Could you check a few things on this drawing? It's one solid part, dimensions in mm from its lowest x, y, z. A direction names the side the tool comes from. Give positions to 0.01 mm unless a question says otherwise; leave off trailing zeros. Loops run counter-clockwise (first coordinate to the right, second up) from the corner with the lowest first, then second, coordinate; pieces in that order, holes last. Notation, with made-up numbers: (-5.5, -7.5) - (45.5, -7.5) arc R23 cw to (45.5, 9.5) - close; hole circle Ø6 at (77, 37.25). An arc over 180 degrees is marked (long way). Return JSON: item names as keys, results as strings. Group by question number.
(1) If we section it at C-C (x = 27.1): Please give me the cut outline in (y, z), then the cut area to 3 significant figures.
(2) For P1, Ø1.5, axis at y = 12, z = 13, coming from the +X side; P2, Ø2.5, axis at y = 10.5, z = 11.5, coming from the +X side; P3, Ø18, axis at x = 63.5, y = 8.5, coming from the +Z side, each with a flat end and sliding along its axis, tell me the tip position at first contact or that it passes through.
(3) If we section it at D-D (z = 6): Please give me the cut outline in (x, y), then the cut area to 3 significant figures.
(4) If we mould it in two halves opening along X, with no side actions, what happens to the marked faces 1, 2 and 3? For each: released by +X, released by -X, zero draft, split by the parting line, or undercut.
(5) If we section it at B-B (z = 13): Please give me the cut outline in (x, y).
(6) On a 3-axis mill with a long thin cutter (end or side, diameter ignored), from which of +Z, -Z, +X, -X, +Y, -Y can I reach the whole of each face in a straight line? I mean the marked faces 4, 5 and 6. Say none if no direction works.
(7) I need wall thicknesses on probe 1 along Y at (x, z) = (27.1, 2.5); probe 2 along X at (y, z) = (5, 12); probe 3 along X at (y, z) = (17, 6.5). Which ranges of each line are inside material? Lowest first, please. Write a range as [from, to].
(8) If we section it at A-A (y = 18): Please give me the cut outline in (x, z), then the cut area to 3 significant figures.
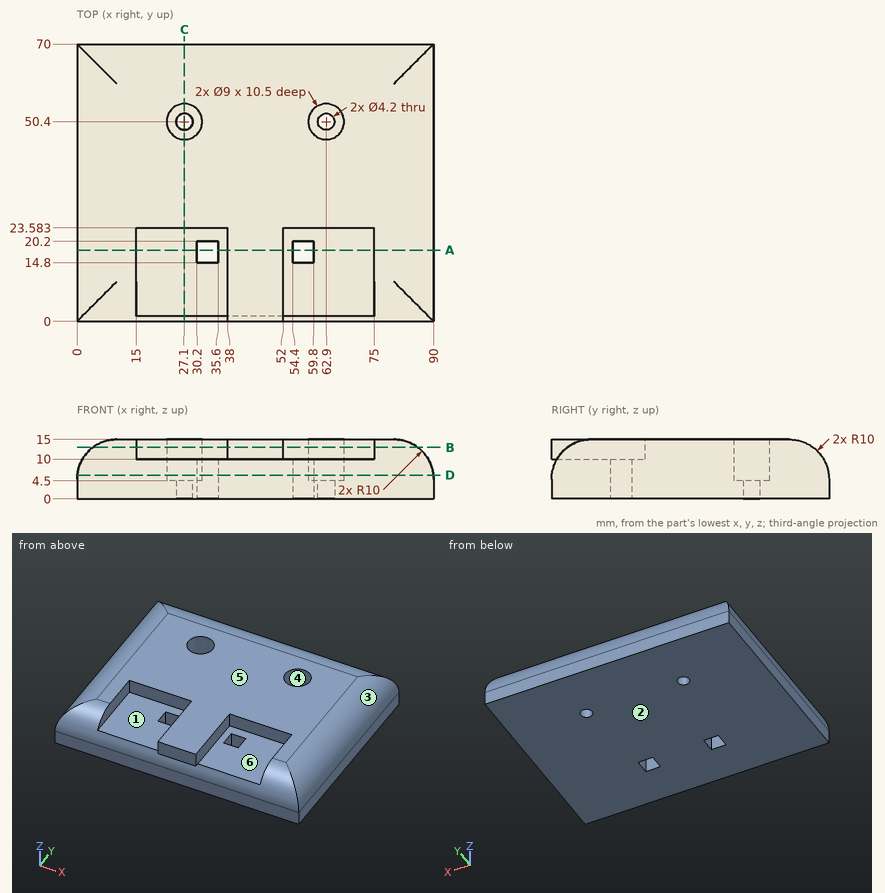
Values:
{
 "1": {"outline": "(0, 0) - (48.3, 0) - (48.3, 4.5) - (45.9, 4.5) - (45.9, 15) - (23.58, 15) - (23.58, 10) - (1.34, 10) arc R10 ccw to (0, 5) - close; (52.5, 0) - (70, 0) - (70, 5) arc R10 ccw to (60, 15) - (54.9, 15) - (54.9, 4.5) - (52.5, 4.5) - close", "area": "795 mm2"},
 "2": {"P1": "x = 86.89", "P2": "x = 88.51", "P3": "z = 10"},
 "3": {"outline": "(0.05, 0.05) - (89.95, 0.05) - (89.95, 69.95) - (0.05, 69.95) - close; hole circle Ø9 at (27.1, 50.4); hole (30.2, 14.8) - (35.6, 14.8) - (35.6, 20.2) - (30.2, 20.2) - close; hole (54.4, 14.8) - (59.8, 14.8) - (59.8, 20.2) - (54.4, 20.2) - close; hole circle Ø9 at (62.9, 50.4)", "area": "6,100 mm2"},
 "4": {"face 1": "undercut", "face 2": "zero draft", "face 3": "released by +X"},
 "5": {"outline": "(4, 4) - (15, 4) - (15, 23.58) - (38, 23.58) - (38, 0) - (52, 0) - (52, 23.58) - (75, 23.58) - (75, 4) - (86, 4) - (86, 66) - (4, 66) - close; hole circle Ø9 at (27.1, 50.4); hole circle Ø9 at (62.9, 50.4)"},
 "6": {"face 4": "+Z", "face 5": "+Z, +X, -X, +Y, -Y", "face 6": "+Z, -Y"},
 "7": {"probe 1": "[0, 48.3], [52.5, 70]", "probe 2": "[2.86, 15], [38, 52], [75, 87.14]", "probe 3": "[0.11, 30.2], [35.6, 54.4], [59.8, 89.89]"},
 "8": {"outline": "(0, 0) - (30.2, 0) - (30.2, 10) - (15, 10) - (15, 15) - (10, 15) arc R10 ccw to (0, 5) - close; (35.6, 0) - (54.4, 0) - (54.4, 10) - (52, 10) - (52, 15) - (38, 15) - (38, 10) - (35.6, 10) - close; (59.8, 0) - (90, 0) - (90, 5) arc R10 ccw to (80, 15) - (75, 15) - (75, 10) - (59.8, 10) - close", "area": "969 mm2"}
}
